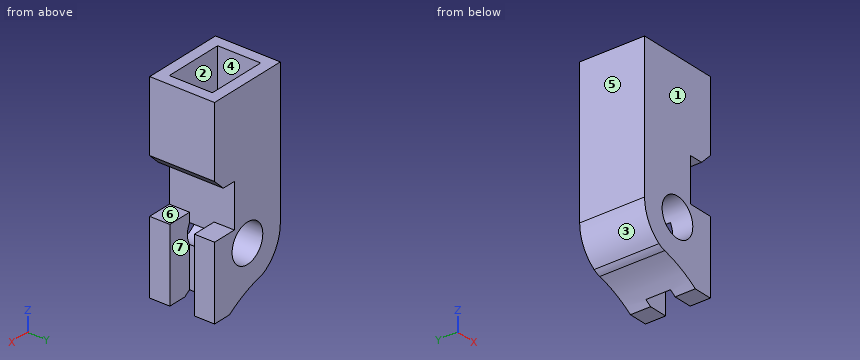
```python
from build123d import *

# Parameters (mm, degrees)
SKETCH3_R               = 3.5
BOSS_EXTRUDE2_DEPTH     = 11.9
CUT_EXTRUDE1_REACH      = 34.374
SKETCH4_W               = 9
SKETCH4_H               = 4.5
SKETCH5_W               = 15
SKETCH5_H               = 11.9
SKETCH5_W_2             = 11
SKETCH5_H_2             = 7.9
BOSS_EXTRUDE3_DEPTH     = 10
CUT_EXTRUDE2_DEPTH      = 33.694142686
CUT_EXTRUDE2_DEPTH_BACK = 33.694142686
SKETCH6_W               = 2.7
SKETCH6_H               = 11.9
CUT_EXTRUDE3_DEPTH      = 31.002615985
CUT_EXTRUDE3_DEPTH_BACK = 31.002615985
FILLET1_R               = 4
CHAMFER1_SIZE           = 2


with BuildPart() as part:
    # Sketch3 → Boss-Extrude2 (new body)
    with BuildSketch(Plane(origin=(0, 0, 0), x_dir=(1, 0, 0), z_dir=(0, 1, 0))):
        with BuildLine():
            Line((7.5, 0), (7.5, 12.657479881))
            Line((7.5, 12.657479881), (4.816081625, 12.657479881))
            ThreePointArc((4.816081625, 12.657479881), (1.359085459, 11.744283435), (-1.195934532, 9.242959169))
            ThreePointArc((-1.195934532, 9.242959169), (-2.208037755, 7.848359435), (-3.45353313, 6.657560283))
            ThreePointArc((-3.45353313, 6.657560283), (-6.40903653, 3.895414068), (-7.5, 0))
            Line((-7.5, 0), (-7.5, -16.500886135))
            Line((-7.5, -16.500886135), (7.5, -16.500886135))
            Line((7.5, -16.500886135), (7.5, -11.500886135))
            Line((7.5, -11.500886135), (3, -11.500886135))
            Line((3, -11.500886135), (3, -3.500886135))
            Line((3, -3.500886135), (7.5, -3.500886135))
            Line((7.5, -3.500886135), (7.5, 0))
        make_face()
        with Locations(Location((0, 0, 0), (0, 0, 270))):
            Circle(SKETCH3_R, mode=Mode.SUBTRACT)
    extrude(amount=BOSS_EXTRUDE2_DEPTH)

    # Cut-Extrude1: up to this face of the body (flat: up to its plane)
    cut_extrude1_end = Plane(part.part.faces().sort_by_distance((5.25, 5.95, 3.500886135))[0])
    # Sketch4 → Cut-Extrude1 (cut, up to the picked face)
    with BuildSketch(Plane(origin=(0, 0, -12.657479881), x_dir=(-1, 0, 0), z_dir=(0, 0, -1)), mode=Mode.PRIVATE) as cut_extrude1_sk1:
        with Locations((-7.5, 5.95)):
            Rectangle(SKETCH4_W, SKETCH4_H)
    cut_extrude1_tool1 = split(extrude(cut_extrude1_sk1.sketch, amount=-CUT_EXTRUDE1_REACH, mode=Mode.PRIVATE), bisect_by=cut_extrude1_end, keep=Keep.BOTH, mode=Mode.PRIVATE)
    add(cut_extrude1_tool1.solids().sort_by(Axis((7.5, 5.95, -12.65748), (0, 0, 1)))[0], mode=Mode.SUBTRACT)

    # Sketch5 → Boss-Extrude3 (add)
    with BuildSketch(Plane.XY.offset(16.500886135)):
        with Locations((0, 5.95)):
            Rectangle(SKETCH5_W, SKETCH5_H)
        with Locations((0, 5.95)):
            Rectangle(SKETCH5_W_2, SKETCH5_H_2, mode=Mode.SUBTRACT)
    extrude(amount=BOSS_EXTRUDE3_DEPTH)

    # Sketch6 → Cut-Extrude2 (cut, two sides: drawn at the far end of the back side and taken through both)
    with BuildSketch(Plane(origin=(7.5, 0, 0), x_dir=(0, 0, -1), z_dir=(1, 0, 0)).offset(-CUT_EXTRUDE2_DEPTH_BACK)):
        with Locations((11.307479881, 5.95)):
            Rectangle(SKETCH6_W, SKETCH6_H)
    extrude(amount=CUT_EXTRUDE2_DEPTH + CUT_EXTRUDE2_DEPTH_BACK, mode=Mode.SUBTRACT)

    # Sketch7 → Cut-Extrude3 (cut, two sides: drawn at the far end of the back side and taken through both)
    with BuildSketch(Plane.XZ.offset(-CUT_EXTRUDE3_DEPTH_BACK)):
        with BuildLine():
            Line((-3.45353313, -6.657560283), (-1.779949015, -9.678496559))
            Line((-1.779949015, -9.678496559), (0.471666332, -11.274565758))
            Line((0.471666332, -11.274565758), (4.067189111, -10.062167039))
            Line((4.067189111, -10.062167039), (4.067189111, -9.957479881))
            ThreePointArc((4.067189111, -9.957479881), (0.471666332, -7.931843239), (-3.45353313, -6.657560283))
        make_face()
    extrude(amount=CUT_EXTRUDE3_DEPTH + CUT_EXTRUDE3_DEPTH_BACK, mode=Mode.SUBTRACT)

    # Fillet1
    fillet1_edges = [part.edges().sort_by_distance(p)[0] for p in [
        (-3.45353313, 5.95, -6.657560283),
    ]]
    fillet(fillet1_edges, radius=FILLET1_R)

    # Chamfer1
    chamfer1_edges = [part.edges().sort_by_distance(p)[0] for p in [
        (7.5, 5.95, 11.500886135),
    ]]
    chamfer(chamfer1_edges, length=CHAMFER1_SIZE)


solid = part.part
```
Here's how the part is built. I have some questions about the finished solid (model axes, mm). Face numbers are marked on the shaded views. A direction names the side the tool comes from. Coordinates: 2 decimals unless noted, no trailing zeros. Write each loop counter-clockwise with the first axis right and the second up, starting at its lowest first coordinate (ties: lowest second). Pieces come first, ordered by that corner, then holes. Notation, with made-up numbers: (58, 86.25) -> (83, 86.25) arc R12 cw to (83, 97.25) -> close; hole circle Ø5 at (82.5, 14.25). An arc over 180 degrees is marked (long way). Use a Markdown table: item, result. Add a question column.
(1) We'd pull the mould along Y, two halves only. Please class the marked faces 1, 2, 3 and 4: +Y half, -Y half, draft (parallel to the pull), parting line (faces both ways), or undercut.
(2) Please list where these lines run through material, in increasing order: line 1 (Z direction, x = 5, y = 10); line 2 (Y direction, x = -1.5, z = 19); line 3 (X direction, y = 2.5, z = 0).
(3) If we section it at A-A, the plane x = 4.75: Write out the boundary of the cut face in (y, z).
(4) For the marked faces 5, 6 and 7, which set-ups out of +Z, -Z, +X, -X, +Y, -Y let a thin tool reach every point of the face, with its end or its side?
(5) If we section it at C-C, the plane x = -2.5: Write out the boundary of the cut face in (y, z).
(6) If we section it at D-D, the plane z = 4: Write out the boundary of the cut face in (x, y).
(7) I'm going to push flat-ended pins straight in: P1, Ø9, axis at x = 0, z = 0, coming from the -Y side; P2, Ø2, axis at x = -5.5, y = 5, coming from the -Z side; P3, Ø3, axis at x = -5, y = 10.5, coming from the -Z side; P4, Ø5, axis at y = 7.5, z = 8.5, coming from the +X side. Where does each tip first touch, or does it pass through?
(8) If we section it at B-B, the plane z = 21: Write out the boundary of the cut face in (x, y), and give its area (3 significant figures).
Outcome:
| question | item | result |
|---|---|---|
| 1 | face 1 | -Y half |
| 1 | face 2 | undercut |
| 1 | face 3 | draft |
| 1 | face 4 | undercut |
| 2 | line 1 | z = -9.96 to 3.5, 11.5 to 26.5 |
| 2 | line 2 | y = 0 to 2, 9.9 to 11.9 |
| 2 | line 3 | x = -7.5 to -3.5, 3.5 to 7.5 |
| 3 | outline | (0, -9.96) -> (3.7, -9.96) -> (3.7, 3.5) -> (0, 3.5) -> close; (0, 11.5) -> (11.9, 11.5) -> (11.9, 26.5) -> (9.9, 26.5) -> (9.9, 16.5) -> (2, 16.5) -> (2, 26.5) -> (0, 26.5) -> close; (8.2, -9.96) -> (11.9, -9.96) -> (11.9, 3.5) -> (8.2, 3.5) -> close |
| 4 | face 5 | +Z, -Z, -X, +Y, -Y |
| 4 | face 6 | +X, +Y, -Y |
| 4 | face 7 | -Z, +X |
| 5 | outline | (0, -6.89) -> (11.9, -6.89) -> (11.9, -2.45) -> (0, -2.45) -> close; (0, 2.45) -> (11.9, 2.45) -> (11.9, 26.5) -> (9.9, 26.5) -> (9.9, 16.5) -> (2, 16.5) -> (2, 26.5) -> (0, 26.5) -> close |
| 6 | outline | (-7.5, 0) -> (3, 0) -> (3, 11.9) -> (-7.5, 11.9) -> close |
| 7 | P1 | stops at y = 0 |
| 7 | P2 | stops at z = -6 |
| 7 | P3 | stops at z = -6.59 |
| 7 | P4 | stops at x = 3 |
| 8 | outline | (-7.5, 0) -> (7.5, 0) -> (7.5, 11.9) -> (-7.5, 11.9) -> close; hole (-5.5, 2) -> (5.5, 2) -> (5.5, 9.9) -> (-5.5, 9.9) -> close |
| 8 | area | 91.6 mm^2 |
